For this review, take the finished solid that the model builds, in its own axes (mm). A direction names the side the tool comes from. Round coordinates to 2 decimals unless told otherwise and drop trailing zeros. Loops run counter-clockwise (first coordinate to the right, second up) from the corner with the lowest first, then second, coordinate; pieces in that order, holes last.
1. Clearance check with flat-ended pins moving along their axes: pin 1 Ø1 at (x, y) = (3.5, 10) entering from +Z; pin 2 Ø2 at (x, y) = (6.5, 7) entering from +Z; pin 3 Ø3 at (y, z) = (14.5, 1.5) entering from +X; pin 4 Ø2 at (x, y) = (9.5, 9) entering from -Z. State where each tip first meets the part, or that it passes through.
2. Consider section D-D on z = 4. State the section outline as (x, y) points, then the cut area to 3 significant figures.
3. Consider section A-A on y = 16. State the section outline as (x, z) points.
4. Consider section C-C on x = 6. State the section outline as (y, z) points, then the cut area to 3 significant figures.
5. Consider section B-B on y = 13.75. State the section outline as (x, z) points.
6. Tool access review of faces 4 (the flat face through (-8, 10, 1.397)), 5 (the flat face through (-6.387, 10, 0)), 6 (the flat face through (-8, 10, -1.603)), 7 (the flat face through (11.613, 10, 0)): name each direction out of +Z, -Z, +X, -X, +Y, -Y from which nothing blocks a thin tool from reaching the whole face with its end or side.
7. To check wall thickness, follow line 1 along X through (y, z) = (6, 0.5); line 2 along Y through (x, z) = (-10, 0.5); line 3 along Z through (x, y) = (9.25, 1.75). State the ranges of each line that lie inside material, in increasing order.
8. Draft analysis for pull direction X (two halves, no side actions). For faces 1 (the flat face through (-1, -1, -5)), 2 (the cylindrical face through (6.67, 10.49, -0.08)), 3 (the flat face through (14.211, -1, 0)), state which applies: released by +X, released by -X, zero draft, split by the parting line, or undercut.
from build123d import *

# Parameters (mm, degrees)
BOSS_EXTRUDE1_DEPTH = 1.5
SKETCH3_W           = 7
SKETCH3_H           = 3
BOSS_EXTRUDE2_DEPTH = 20
SKETCH4_R           = 1.705
CUT_EXTRUDE1_DEPTH  = 5
LPATTERN1_COUNT     = 3
LPATTERN1_PITCH     = 5


with BuildPart() as part:
    # Sketch1 → Boss-Extrude1 (new body)
    with BuildSketch(Plane(origin=(0, 0, 0), x_dir=(1, 0, 0), z_dir=(0, 1, 0))):
        Polygon((-5.789473684, 5), (-15.789473684, 5), (-15.789473684, -5), (-5.789473684, -5), (4.210526316, -5), (14.210526316, -5), (14.210526316, 5), (4.210526316, 5), align=None)
    extrude(amount=-BOSS_EXTRUDE1_DEPTH)

    # Sketch3 → Boss-Extrude2 (add)
    with BuildSketch(Plane(origin=(0, 0, 0), x_dir=(1, 0, 0), z_dir=(0, 1, 0))):
        with Locations((-9.886735186, 0.10262718)):
            Rectangle(SKETCH3_W, SKETCH3_H)
        with Locations((8.113264814, 0.10262718)):
            Rectangle(SKETCH3_W, SKETCH3_H)
    extrude(amount=BOSS_EXTRUDE2_DEPTH)

    # Sketch4 → Cut-Extrude1 (cut, symmetric)
    with BuildSketch(Plane.XY):
        with Locations(Location((-10.0595209, 16, 0), (0, 0, 180))):
            Circle(SKETCH4_R)
        with Locations(Location((8.29517143, 16, 0), (0, 0, 180))):
            Circle(SKETCH4_R)
    cut_extrude1 = extrude(amount=CUT_EXTRUDE1_DEPTH, both=True, mode=Mode.SUBTRACT)

    # LPattern1: Cut-Extrude1 ×3
    with Locations(*[(0, -i * LPATTERN1_PITCH, 0) for i in range(1, LPATTERN1_COUNT)]):
        add(cut_extrude1, mode=Mode.SUBTRACT)


solid = part.part
Resolved:
1. pin 1: passes through
1. pin 2: stops at z = 1.4
1. pin 3: stops at x = 11.61
1. pin 4: stops at z = -1.6
2. outline: (-15.79, -1.5) - (14.21, -1.5) - (14.21, 0) - (-15.79, 0) - close
2. area: 45.0 mm2
3. outline: (-13.39, -1.6) - (-11.76, -1.6) - (-11.76, 1.4) - (-13.39, 1.4) - close; (-8.35, -1.6) - (-6.39, -1.6) - (-6.39, 1.4) - (-8.35, 1.4) - close; (4.61, -1.6) - (6.59, -1.6) - (6.59, 1.4) - (4.61, 1.4) - close; (10, -1.6) - (11.61, -1.6) - (11.61, 1.4) - (10, 1.4) - close
4. outline: (-1.5, -5) - (0, -5) - (0, -1.6) - (20, -1.6) - (20, 1.4) - (0, 1.4) - (0, 5) - (-1.5, 5) - close
4. area: 75.0 mm2
5. outline: (-13.39, -1.6) - (-6.39, -1.6) - (-6.39, 1.4) - (-13.39, 1.4) - close; (4.61, -1.6) - (11.61, -1.6) - (11.61, 1.4) - (4.61, 1.4) - close
6. face 4: +Z, +X, -X, +Y
6. face 5: +Z, -Z, +Y
6. face 6: -Z, +X, -X, +Y
6. face 7: +Z, -Z, +X, +Y
7. line 1: x = -13.39 to -11.76, -8.35 to -6.39, 4.61 to 6.59, 10 to 11.61
7. line 2: y = -1.5 to 4.3, 7.7 to 9.3, 12.7 to 14.3, 17.7 to 20
7. line 3: z = -1.6 to 1.4
8. face 1: zero draft
8. face 2: undercut
8. face 3: released by +X
